Here's how the part is built. I have some questions about the finished solid (model axes, mm). Face numbers are marked on the shaded views. A direction names the side the tool comes from. Coordinates: 2 decimals unless noted, no trailing zeros. Order: outer loops, then holes, each group sorted by start corner. A loop starts at its lowest first (then second) coordinate and runs counter-clockwise, first axis right, second up. Notation, with made-up numbers: (79.5, 43) - (94.5, 43) arc R19 ccw to (94.5, 72) - close; hole circle Ø9 at (-21.75, 11.25). An arc over 180 degrees is marked (long way). Answer as CSV lines item,"result". Start each with the question number.
Q1. Suppose I cut it at A-A (z = 19.05). Please give me the cut outline in (x, y) (1 decimal), then the cut area to 3 significant figures.
Q2. For pin 1 Ø1.9 at (y, z) = (5, -22.5) entering from +X; pin 2 Ø4 at (x, z) = (22.225, 19.05) entering from +Y; pin 3 Ø1 at (x, z) = (-6, 9.5) entering from +Y (3 decimals); pin 4 Ø3 at (x, z) = (4, -22) entering from -Y, each with a flat end and sliding along its axis, tell me the tip position at first contact or that it passes through.
Q3. Suppose I cut it at C-C (y = -6.5). Count the separate pieces of the cut face and the enclosed holes in it, then the cut area to 3 significant figures.
Q4. I need wall thicknesses on line 1 (Y direction, x = -15, z = 0.5) (3 decimals); line 2 (Y direction, x = 15.5, z = -20.5) (3 decimals); line 3 (Z direction, x = -3, y = -20.5) (3 decimals). Which ranges of each line are inside material? Lowest first, please.
Q5. For the marked faces 1 and 2, which set-ups out of +Z, -Z, +X, -X, +Y, -Y let a thin tool reach every point of the face, with its end or its side?
Q6. Suppose I cut it at B-B (y = 4). Please give me the cut outline in (x, z) (1 decimal).
from build123d import *

# Parameters (mm, degrees)
SKETCH1_R           = 2.2225
BOSS_EXTRUDE1_DEPTH = 1.905
SKETCH2_W           = 1.27
SKETCH2_H           = 31.75
SKETCH2_W_2         = 1.228725
BOSS_EXTRUDE2_DEPTH = 28.575
SKETCH3_W           = 1.228725
SKETCH3_H           = 1.905
BOSS_EXTRUDE4_DEPTH = 31.75
SKETCH4_W           = 17.78
SKETCH4_H           = 5.08
BOSS_EXTRUDE5_DEPTH = 6.35
CUT_EXTRUDE1_DEPTH  = 19.05
SKETCH6_R           = 1.27
CUT_EXTRUDE2_DEPTH  = 3.175
SKETCH7_W           = 2.54
SKETCH7_H           = 4.445
CUT_EXTRUDE3_DEPTH  = 4.445


with BuildPart() as part:
    # Sketch1 → Boss-Extrude1 (new body)
    with BuildSketch(Plane(origin=(0, 0, 0), x_dir=(1, 0, 0), z_dir=(0, 1, 0))):
        Polygon((-21.59, 25.4), (-25.4, 21.59), (-25.4, -21.59), (-21.59, -25.4), (21.59, -25.4), (25.4, -21.59), (25.4, 21.59), (21.59, 25.4), align=None)
        with Locations(Location((-22.225, 19.05, 0), (0, 0, 90))):
            Circle(SKETCH1_R, mode=Mode.SUBTRACT)
        with Locations(Location((22.225, 19.05, 0), (0, 0, 90))):
            Circle(SKETCH1_R, mode=Mode.SUBTRACT)
        with Locations(Location((22.225, -19.05, 0), (0, 0, 90))):
            Circle(SKETCH1_R, mode=Mode.SUBTRACT)
        with Locations(Location((-22.225, -19.05, 0), (0, 0, 90))):
            Circle(SKETCH1_R, mode=Mode.SUBTRACT)
    extrude(amount=BOSS_EXTRUDE1_DEPTH)

    # Sketch2 → Boss-Extrude2 (add)
    with BuildSketch(Plane.XZ):
        with Locations((-24.765, 0)):
            Rectangle(SKETCH2_W, SKETCH2_H)
        with Locations((-21.6487375, 0)):
            Rectangle(SKETCH2_W_2, SKETCH2_H)
        with Locations((-18.5531125, 0)):
            Rectangle(SKETCH2_W_2, SKETCH2_H)
        with Locations((-15.4574875, 0)):
            Rectangle(SKETCH2_W_2, SKETCH2_H)
        with Locations((-12.3618625, 0)):
            Rectangle(SKETCH2_W_2, SKETCH2_H)
        with Locations((-9.2662375, 0)):
            Rectangle(SKETCH2_W_2, SKETCH2_H)
        with Locations((-6.1706125, 0)):
            Rectangle(SKETCH2_W_2, SKETCH2_H)
        with Locations((-3.0749875, 0)):
            Rectangle(SKETCH2_W_2, SKETCH2_H)
        with Locations((0.0206375, 0)):
            Rectangle(SKETCH2_W_2, SKETCH2_H)
        with Locations((3.1162625, 0)):
            Rectangle(SKETCH2_W_2, SKETCH2_H)
        with Locations((6.2118875, 0)):
            Rectangle(SKETCH2_W_2, SKETCH2_H)
        with Locations((9.3075125, 0)):
            Rectangle(SKETCH2_W_2, SKETCH2_H)
        with Locations((12.4031375, 0)):
            Rectangle(SKETCH2_W_2, SKETCH2_H)
        with Locations((15.4987625, 0)):
            Rectangle(SKETCH2_W_2, SKETCH2_H)
        with Locations((18.5943875, 0)):
            Rectangle(SKETCH2_W_2, SKETCH2_H)
        with Locations((21.6900125, 0)):
            Rectangle(SKETCH2_W_2, SKETCH2_H)
        with Locations((24.7856375, 0)):
            Rectangle(SKETCH2_W_2, SKETCH2_H)
    extrude(amount=BOSS_EXTRUDE2_DEPTH)

    # Sketch3 → Boss-Extrude4 (add)
    with BuildSketch(Plane.XY.offset(15.875)):
        with BuildLine():
            Line((-19.167475, 0), (-24.13, 0))
            Line((-24.13, 0), (-24.13, -1.905))
            ThreePointArc((-24.13, -1.905), (-23.19655, -0.97155), (-22.2631, -1.905))
            Line((-22.2631, -1.905), (-21.034375, -1.905))
            ThreePointArc((-21.034375, -1.905), (-20.100925, -0.97155), (-19.167475, -1.905))
            Line((-19.167475, -1.905), (-19.167475, 0))
        make_face()
        with BuildLine():
            Line((24.171275, 0), (-17.93875, 0))
            Line((-17.93875, 0), (-17.93875, -1.905))
            ThreePointArc((-17.93875, -1.905), (-17.0053, -0.97155), (-16.07185, -1.905))
            Line((-16.07185, -1.905), (-14.843125, -1.905))
            ThreePointArc((-14.843125, -1.905), (-13.909675, -0.97155), (-12.976225, -1.905))
            Line((-12.976225, -1.905), (-11.7475, -1.905))
            ThreePointArc((-11.7475, -1.905), (-10.81405, -0.97155), (-9.8806, -1.905))
            Line((-9.8806, -1.905), (-8.651875, -1.905))
            ThreePointArc((-8.651875, -1.905), (-7.718425, -0.97155), (-6.784975, -1.905))
            Line((-6.784975, -1.905), (-5.55625, -1.905))
            ThreePointArc((-5.55625, -1.905), (-4.6228, -0.97155), (-3.68935, -1.905))
            Line((-3.68935, -1.905), (-2.460625, -1.905))
            ThreePointArc((-2.460625, -1.905), (-1.527175, -0.97155), (-0.593725, -1.905))
            Line((-0.593725, -1.905), (0.635, -1.905))
            ThreePointArc((0.635, -1.905), (1.56845, -0.97155), (2.5019, -1.905))
            Line((2.5019, -1.905), (3.730625, -1.905))
            ThreePointArc((3.730625, -1.905), (4.664075, -0.97155), (5.597525, -1.905))
            Line((5.597525, -1.905), (6.82625, -1.905))
            ThreePointArc((6.82625, -1.905), (7.7597, -0.97155), (8.69315, -1.905))
            Line((8.69315, -1.905), (9.921875, -1.905))
            ThreePointArc((9.921875, -1.905), (10.855325, -0.97155), (11.788775, -1.905))
            Line((11.788775, -1.905), (13.0175, -1.905))
            ThreePointArc((13.0175, -1.905), (13.95095, -0.97155), (14.8844, -1.905))
            Line((14.8844, -1.905), (16.113125, -1.905))
            ThreePointArc((16.113125, -1.905), (17.046575, -0.97155), (17.980025, -1.905))
            Line((17.980025, -1.905), (19.20875, -1.905))
            ThreePointArc((19.20875, -1.905), (20.1422, -0.97155), (21.07565, -1.905))
            Line((21.07565, -1.905), (22.304375, -1.905))
            ThreePointArc((22.304375, -1.905), (23.237825, -0.97155), (24.171275, -1.905))
            Line((24.171275, -1.905), (24.171275, 0))
        make_face()
        with Locations((-18.5531125, -0.9525)):
            Rectangle(SKETCH3_W, SKETCH3_H)
    extrude(amount=-BOSS_EXTRUDE4_DEPTH)

    # Sketch4 → Boss-Extrude5 (add)
    with BuildSketch(Plane(origin=(0, 1.905, 0), x_dir=(1, 0, 0), z_dir=(0, 1, 0))):
        with Locations((6.6675, 22.225)):
            Rectangle(SKETCH4_W, SKETCH4_H)
    extrude(amount=BOSS_EXTRUDE5_DEPTH)

    # Sketch5 → Cut-Extrude1 (cut)
    with BuildSketch(Plane(origin=(15.5575, 0, 0), x_dir=(0, 0, -1), z_dir=(1, 0, 0))):
        Polygon((19.685, 8.255), (19.685, 1.905), (20.32, 8.255), align=None)
        Polygon((24.765, 8.255), (24.13, 8.255), (24.765, 1.905), align=None)
    extrude(amount=-CUT_EXTRUDE1_DEPTH, mode=Mode.SUBTRACT)

    # Sketch6 → Cut-Extrude2 (cut)
    with BuildSketch(Plane(origin=(0, 8.255, 0), x_dir=(1, 0, 0), z_dir=(0, 1, 0))):
        with Locations(Location((-0.3175, 22.225, 0), (0, 0, 270))):
            Circle(SKETCH6_R)
        with Locations(Location((4.339166667, 22.225, 0), (0, 0, 270))):
            Circle(SKETCH6_R)
        with Locations(Location((8.995833333, 22.225, 0), (0, 0, 270))):
            Circle(SKETCH6_R)
        with Locations(Location((13.6525, 22.225, 0), (0, 0, 270))):
            Circle(SKETCH6_R)
    extrude(amount=-CUT_EXTRUDE2_DEPTH, mode=Mode.SUBTRACT)

    # Sketch7 → Cut-Extrude3 (cut)
    with BuildSketch(Plane(origin=(0, 0, -25.4), x_dir=(-1, 0, 0), z_dir=(0, 0, -1))):
        with Locations((-13.335, 5.08)):
            Rectangle(SKETCH7_W, SKETCH7_H)
        with Locations((-8.89, 5.08)):
            Rectangle(SKETCH7_W, SKETCH7_H)
        with Locations((-4.445, 5.08)):
            Rectangle(SKETCH7_W, SKETCH7_H)
        with Locations((0, 5.08)):
            Rectangle(SKETCH7_W, SKETCH7_H)
    extrude(amount=-CUT_EXTRUDE3_DEPTH, mode=Mode.SUBTRACT)


solid = part.part
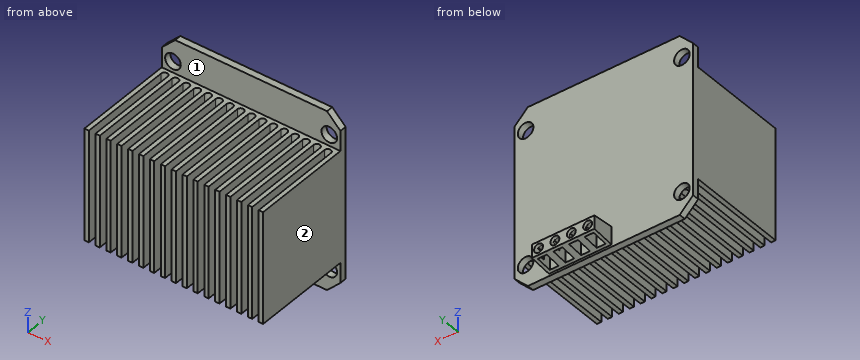
Here are the results:
1,outline,"(-25.4, 0) - (-24.4, 0) - (-24.4, 1.9) - (-25.4, 1.9) - close; (-20, 0) - (20, 0) - (20, 1.9) - (-20, 1.9) - close; (24.4, 0) - (25.4, 0) - (25.4, 1.9) - (24.4, 1.9) - close"
1,area,"79.8 mm²"
2,pin 1,"stops at x = 15.56"
2,pin 2,"passes through"
2,pin 3,"stops at y = 1.905"
2,pin 4,"stops at y = 0"
3,separate pieces,"17"
3,enclosed holes,"0"
3,area,"665 mm²"
4,line 1,"y = -28.575 to 1.905"
4,line 2,"y = 0 to 8.255"
4,line 3,"z = -15.875 to 15.875"
5,face 1,"+Z, +X, -X, -Y"
5,face 2,"+Z, -Z, +X, +Y, -Y"
6,outline,"(-2.2, -24.6) - (-1.3, -24.6) - (-1.3, -21) - (1.3, -21) - (1.3, -24.6) - (3.2, -24.6) - (3.2, -21) - (5.7, -21) - (5.7, -24.6) - (7.6, -24.6) - (7.6, -21) - (10.2, -21) - (10.2, -24.6) - (12.1, -24.6) - (12.1, -21) - (14.6, -21) - (14.6, -24.6) - (15.6, -24.6) - (15.6, -19.9) - (-2.2, -19.9) - close"
